Work out the finished part from the listing and answer in its coordinate system (mm). Face numbers are marked on the shaded views. A direction names the side the tool comes from. Round coordinates to 2 decimals unless told otherwise and drop trailing zeros. Write each loop counter-clockwise with the first axis right and the second up, starting at its lowest first coordinate (ties: lowest second). Pieces come first, ordered by that corner, then holes. Notation, with made-up numbers: (-31, -30.5) - (-16, -30.5) arc R18 cw to (-16, -5.5) - close; hole circle Ø6 at (24.5, 52). An arc over 180 degrees is marked (long way). Answer as a JSON object with one key per item and string values.
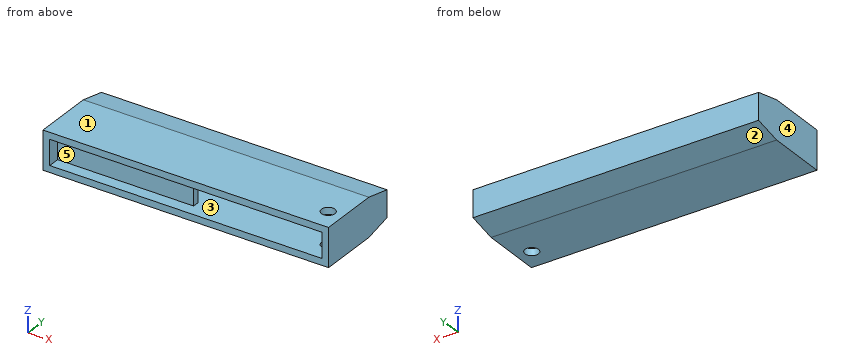
```python
from build123d import *

# Parameters (mm, degrees)
BOSS_EXTRUDE1_DEPTH      = 8
BOSS_EXTRUDE1_DEPTH_BACK = 17.8
SKETCH1_W                = 138
SKETCH1_H                = 11.5
SKETCH8_R                = 2
CUT_EXTRUDE4_DEPTH       = 11.5
CHAMFER2_SIZE            = 8
CHAMFER2_SIZE2           = 1.75
CHAMFER3_SIZE            = 1.75
CHAMFER3_SIZE2           = 8
CUT_EXTRUDE5_REACH       = 75.89
SKETCH11_W               = 53
SKETCH11_H               = 11.5
SKETCH12_W               = 81
SKETCH12_H               = 7.5
CUT_EXTRUDE6_DEPTH       = 17.8
SKETCH13_W               = 40.5
SKETCH13_H               = 2
BOSS_EXTRUDE3_DEPTH      = 7.5


with BuildPart() as part:
    # Sketch1 → Boss-Extrude1 (new, two sides: drawn at the far end of the back side and taken through both)
    with BuildSketch(Plane(origin=(0, 0, 0), x_dir=(1, 0, 0), z_dir=(0, 1, 0)).offset(-BOSS_EXTRUDE1_DEPTH_BACK)):
        Rectangle(SKETCH1_W, SKETCH1_H)
    extrude(amount=BOSS_EXTRUDE1_DEPTH + BOSS_EXTRUDE1_DEPTH_BACK)

    # Sketch8 → Cut-Extrude4 (cut)
    with BuildSketch(Plane.XY.offset(5.75)):
        with Locations((64.55, -11.35)):
            Circle(SKETCH8_R)
    extrude(amount=-CUT_EXTRUDE4_DEPTH, mode=Mode.SUBTRACT)

    # Chamfer2
    chamfer2_edges = [part.edges().sort_by_distance(p)[0] for p in [
        (0, 8, 5.75),
    ]]
    chamfer2_side = [part.faces().sort_by_distance(p)[0] for p in [
        (-0.228635079, -4.877154202, 5.75),
    ]]
    chamfer(chamfer2_edges, length=CHAMFER2_SIZE, length2=CHAMFER2_SIZE2, reference=chamfer2_side[0])

    # Chamfer3
    chamfer3_edges = [part.edges().sort_by_distance(p)[0] for p in [
        (0, 8, -5.75),
    ]]
    chamfer3_side = [part.faces().sort_by_distance(p)[0] for p in [
        (0, 8, -0.875),
    ]]
    chamfer(chamfer3_edges, length=CHAMFER3_SIZE, length2=CHAMFER3_SIZE2, reference=chamfer3_side[0])

    # Cut-Extrude5: up to this face of the body (flat: up to its plane)
    cut_extrude5_end = Plane(part.part.faces().sort_by_distance((0, 8, 0))[0])
    # Sketch11 → Cut-Extrude5 (cut, up to the picked face)
    with BuildSketch(Plane.XZ.offset(17.8), mode=Mode.PRIVATE) as cut_extrude5_sk1:
        with Locations((-42.5, 0)):
            Rectangle(SKETCH11_W, SKETCH11_H)
    cut_extrude5_tool1 = split(extrude(cut_extrude5_sk1.sketch, amount=-CUT_EXTRUDE5_REACH, mode=Mode.PRIVATE), bisect_by=cut_extrude5_end, keep=Keep.BOTH, mode=Mode.PRIVATE)
    add(cut_extrude5_tool1.solids().sort_by(Axis((-42.5, -17.8, 0), (0, 1, 0)))[0], mode=Mode.SUBTRACT)

    # Sketch12 → Cut-Extrude6 (cut)
    with BuildSketch(Plane.XZ.offset(17.8)):
        with Locations((26.5, 0)):
            Rectangle(SKETCH12_W, SKETCH12_H)
    extrude(amount=-CUT_EXTRUDE6_DEPTH, mode=Mode.SUBTRACT)

    # Sketch13 → Boss-Extrude3 (add)
    with BuildSketch(Plane.XY.offset(-3.75)):
        with Locations((6.25, -13.3)):
            Rectangle(SKETCH13_W, SKETCH13_H)
    extrude(amount=BOSS_EXTRUDE3_DEPTH)


solid = part.part
```
Item 1: A cutting plane is placed at D-D (y = -5.25). Write down the section's boundary in (x, z).
Results found:
{"outline": "(-16, -5.75) - (69, -5.75) - (69, 5.75) - (-16, 5.75) - close; hole (-14, -3.75) - (67, -3.75) - (67, 3.75) - (-14, 3.75) - close"}
Item 2: For the marked faces 4 and 5, determine the directions among +Z, -Z, +X, -X, +Y, -Y from which every point of the face is accessible in a straight line to the end or side of a thin tool.
Results found:
{"face 4": "+Z, -Z, -X, +Y, -Y", "face 5": "-Y"}
Item 3: A cutting plane is placed at A-A (x = 64.55). Write down the section's boundary in (y, z), and give its area (3 significant figures).
Results found:
{"outline": "(-17.8, -5.75) - (-13.35, -5.75) - (-13.35, -3.75) - (-17.8, -3.75) - close; (-17.8, 3.75) - (-13.35, 3.75) - (-13.35, 5.75) - (-17.8, 5.75) - close; (-9.35, -5.75) - (0, -5.75) - (8, -4) - (8, 4) - (0, 5.75) - (-9.35, 5.75) - (-9.35, 3.75) - (0, 3.75) - (0, -3.75) - (-9.35, -3.75) - close", "area": "133 mm²"}
Item 4: A cutting plane is placed at B-B (y = -11.35). Write down the section's boundary in (x, z).
Results found:
{"outline": "(-16, -5.75) - (62.55, -5.75) - (62.55, -3.75) - (-14, -3.75) - (-14, 3.75) - (62.55, 3.75) - (62.55, 5.75) - (-16, 5.75) - close; (66.55, -5.75) - (69, -5.75) - (69, 5.75) - (66.55, 5.75) - (66.55, 3.75) - (67, 3.75) - (67, -3.75) - (66.55, -3.75) - close"}
Item 5: Each of these flat-tipped pins is pushed along its axis until it touches: P1, Ø3.5, axis at x = 64.55, y = -11.35, coming from the -Z side; P2, Ø1, axis at x = 56, z = -0.5, coming from the -Y side; P3, Ø5, axis at x = 11.5, z = 2.5, coming from the -Y side. Where does it stop, or does it pass through?
Results found:
{"P1": "through", "P2": "y = 0", "P3": "y = -17.8"}
Item 6: A cutting plane is placed at C-C (x = -6). Write down the section's boundary in (y, z), and give its area (3 significant figures).
Results found:
{"outline": "(-17.8, -5.75) - (0, -5.75) - (8, -4) - (8, 4) - (0, 5.75) - (-17.8, 5.75) - (-17.8, 3.75) - (-14.3, 3.75) - (-14.3, -3.75) - (-17.8, -3.75) - close; hole (-12.3, -3.75) - (0, -3.75) - (0, 3.75) - (-12.3, 3.75) - close", "area": "164 mm²"}
Item 7: Determine the mould class of the marked faces 1, 2 and 3 for opening direction Y: pulls with the +Y half, pulls with the -Y half, needs draft (parallel to the pull), parting line crosses it, or undercut.
Results found:
{"face 1": "needs draft", "face 2": "pulls with the +Y half", "face 3": "undercut"}
Item 8: Consider line 1 along Z through (x, y) = (62.5, -4); line 2 along Y through (x, z) = (11, -2.5); line 3 along X through (y, z) = (-4.25, 0.75). Determine where each line is inside the solid, lowest interval first.
Results found:
{"line 1": "-5.75 to -3.75, 3.75 to 5.75", "line 2": "-14.3 to -12.3, 0 to 8", "line 3": "-16 to -14, 67 to 69"}
